Drawing for the job (mm, zero at the part's lowest x, y, z). A direction names the side the tool comes from. Give positions to 0.01 mm unless a question says otherwise; leave off trailing zeros. Write each loop counter-clockwise with the first axis right and the second up, starting at its lowest first coordinate (ties: lowest second). Pieces come first, ordered by that corner, then holes.
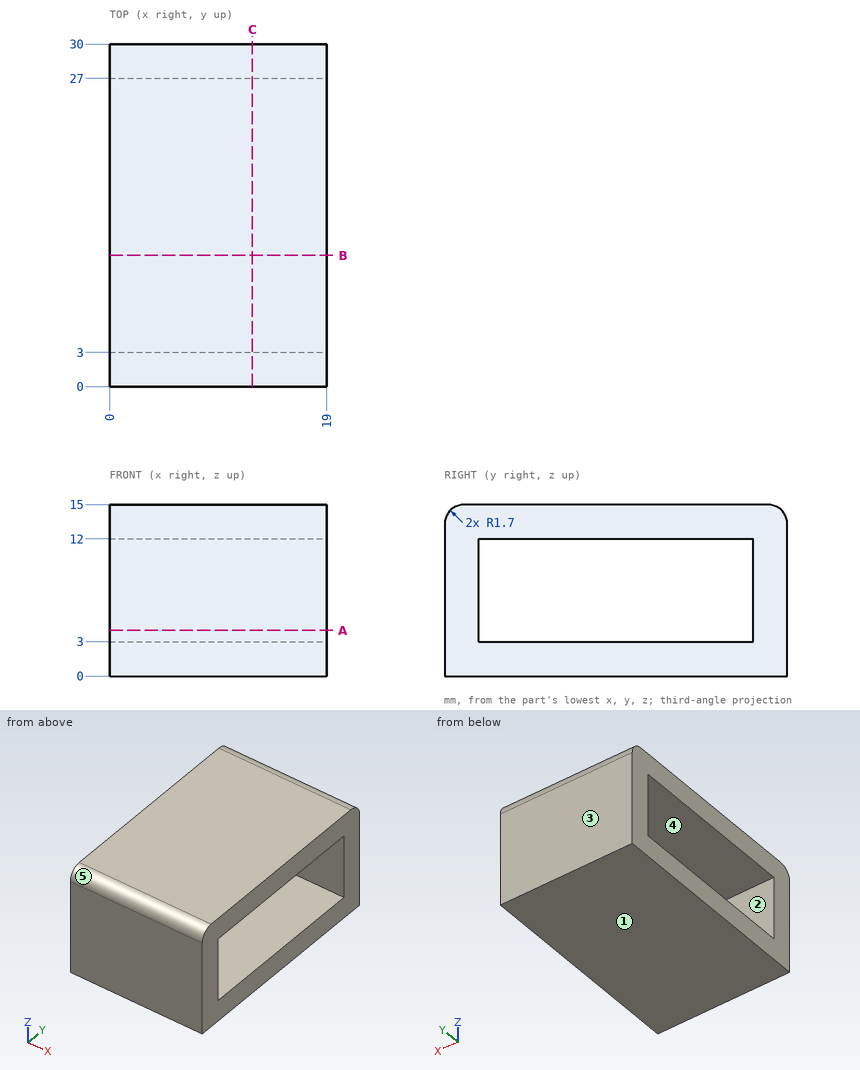
1. Probe probe 1 along Z at (x, y) = (4, 11.5); probe 2 along Y at (x, z) = (16.25, 11.25); probe 3 along Z at (x, y) = (2, 29.5). List the from-to ranges inside material, lowest first.
Calculated:
probe 1: z = 0 to 3, 12 to 15
probe 2: y = 0 to 3, 27 to 30
probe 3: z = 0 to 14.5
2. Pull direction Z, two halves, no side cores. Call the marked faces 3, 4 and 5: +Z half, -Z half, draft (parallel to the pull), parting line (faces both ways), or undercut.
Calculated:
face 3: draft
face 4: undercut
face 5: +Z half
3. Slice it at B-B, the plane y = 11.5. Write the cut outline in (x, z), and give its area (3 significant figures).
Calculated:
outline: (0, 0) - (19, 0) - (19, 3) - (0, 3) - close; (0, 12) - (19, 12) - (19, 15) - (0, 15) - close
area: 114 mm2
4. Slice it at C-C, the plane x = 12.5. Write the cut outline in (y, z), and give its area (3 significant figures).
Calculated:
outline: (0, 0) - (30, 0) - (30, 13.3) arc R1.7 ccw to (28.3, 15) - (1.7, 15) arc R1.7 ccw to (0, 13.3) - close; hole (3, 3) - (27, 3) - (27, 12) - (3, 12) - close
area: 233 mm2
5. Which spindle directions (+Z, -Z, +X, -X, +Y, -Y) get a long thin tool onto all of the face, cutting with end or side? Do the marked faces 1 and 2. Say none if no direction does.
Calculated:
face 1: -Z, +X, -X, +Y, -Y
face 2: +X, -X
6. Slice it at A-A, the plane z = 4. Write the cut outline in (x, y).
Calculated:
outline: (0, 0) - (19, 0) - (19, 3) - (0, 3) - close; (0, 27) - (19, 27) - (19, 30) - (0, 30) - close
